```python
from build123d import *

# Parameters (mm, degrees)
CROQUIS1_W              = 102
CROQUIS1_H              = 70
SALIENTE_EXTRUIR1_DEPTH = 24
CROQUIS2_W              = 98
CROQUIS2_H              = 66
CORTAR_EXTRUIR1_DEPTH   = 21
CORTAR_EXTRUIR2_DEPTH   = 2


with BuildPart() as part:
    # Croquis1 → Saliente-Extruir1 (new body)
    with BuildSketch(Plane(origin=(0, 0, 0), x_dir=(1, 0, 0), z_dir=(0, 1, 0))):
        with Locations((51, 35)):
            Rectangle(CROQUIS1_W, CROQUIS1_H)
    extrude(amount=SALIENTE_EXTRUIR1_DEPTH)

    # Croquis2 → Cortar-Extruir1 (cut)
    with BuildSketch(Plane(origin=(0, 24, 0), x_dir=(1, 0, 0), z_dir=(0, 1, 0))):
        with Locations((51, 35)):
            Rectangle(CROQUIS2_W, CROQUIS2_H)
    extrude(amount=-CORTAR_EXTRUIR1_DEPTH, mode=Mode.SUBTRACT)

    # Croquis3 → Cortar-Extruir2 (cut)
    with BuildSketch(Plane(origin=(102, 0, 0), x_dir=(0, 0, -1), z_dir=(1, 0, 0))):
        Polygon((6, 9), (60, 9), (60, 10.8), (57.25, 10.8), (57.25, 22.3), (47.75, 22.3), (47.75, 19.6), (38.75, 19.6), (38.75, 10.8), (26.75, 10.8), (26.75, 19.3), (11.75, 19.3), (11.75, 10.8), (6, 10.8), align=None)
    extrude(amount=-CORTAR_EXTRUIR2_DEPTH, mode=Mode.SUBTRACT)


solid = part.part
```
Geometry check sheet. Reference: the model listing, model coordinates, mm. A direction names the side the tool comes from. Coordinates: 2 decimals unless noted, no trailing zeros. Order: outer loops, then holes, each group sorted by start corner. A loop starts at its lowest first (then second) coordinate and runs counter-clockwise, first axis right, second up. Notation, with made-up numbers: (50.25, 89.25) - (99.25, 89.25) arc R23 ccw to (99.25, 102.25) - close; hole circle Ø9 at (-3, 53.5). An arc over 180 degrees is marked (long way). Use one line per item in the form item = value.
1. Access from +Z, -Z, +X, -X, +Y, -Y to the whole of each face (thin tool, end or side, straight path). Record for faces 1 (the face through (0, 12, -35)), 2 (the face through (50, 14, -68)), 3 (the face through (101, 16, -57.25)).
Here are the results:
face_1 = +Z, -Z, -X, +Y, -Y
face_2 = +Y
face_3 = +X
2. Gauge pin test, flat end, axial feed: pin 1 (20 mm diameter, centred on x = 46, z = -47.5, fed in from +Y). Record the tip position at first contact, or that the pin passes through.
Here are the results:
pin_1 = 3
3. Section check A-A (y = 16.25). Record the boundary of the cut face in (x, z).
Here are the results:
outline = (0, -70) - (102, -70) - (102, -57.25) - (100, -57.25) - (100, -68) - (2, -68) - (2, -2) - (100, -2) - (100, -11.75) - (102, -11.75) - (102, 0) - (0, 0) - close; (100, -38.75) - (102, -38.75) - (102, -26.75) - (100, -26.75) - close
4. Section check B-B (z = -46). Record the boundary of the cut face in (x, y).
Here are the results:
outline = (0, 0) - (102, 0) - (102, 9) - (100, 9) - (100, 3) - (2, 3) - (2, 24) - (0, 24) - close; (100, 19.6) - (102, 19.6) - (102, 24) - (100, 24) - close
5. Scan lines: line 1 (X direction, y = 12.75, z = -32); line 2 (Z direction, x = 76, y = 20.75); line 3 (Y direction, x = 82.5, z = -19). Record each from-to range of solid material in increasing order.
Here are the results:
line_1 = 0 to 2, 100 to 102
line_2 = -70 to -68, -2 to 0
line_3 = 0 to 3
6. Section check D-D (x = 76). Record the boundary of the cut face in (y, z), then the cut area to 3 significant figures.
Here are the results:
outline = (0, -70) - (24, -70) - (24, -68) - (3, -68) - (3, -2) - (24, -2) - (24, 0) - (0, 0) - close
area = 294 mm²
7. Section check C-C (y = 7.5). Record the boundary of the cut face in (x, z), then the cut area to 3 significant figures.
Here are the results:
outline = (0, -70) - (102, -70) - (102, 0) - (0, 0) - close; hole (2, -68) - (100, -68) - (100, -2) - (2, -2) - close
area = 672 mm²
8. Draft check along Z on faces 4 (the face through (50, 0, -35)), 5 (the face through (50, 12, -70)), 6 (the face through (101, 10.8, -33)). Enter one of: pulls with the +Z half, pulls with the -Z half, needs draft (parallel to the pull), parting line crosses it, or undercut.
Here are the results:
face_4 = needs draft
face_5 = pulls with the -Z half
face_6 = undercut
